from build123d import *

# Parameters (mm, degrees)
F0_W      = 78.3574953675
F0_H      = 53.3467046916
F1_DEPTH  = 50.8
F3_DEPTH  = 50.801
F4_W      = 25.4
F4_H      = 40.6467046916
F5_DEPTH  = 50.801
F6_W      = 12.7
F6_H      = 12.7
F7_DEPTH  = 50.801
F9_DEPTH  = 12.7
F11_DEPTH = 12.7
F13_DEPTH = 78.3584953675
F14_R     = 6.35


with BuildPart() as f1:
    # F0 (on Front) → F1 (new body)
    with BuildSketch(Plane.XZ):
        with Locations((39.1787476838, 26.6733523458)):
            Rectangle(F0_W, F0_H)
    extrude(amount=-F1_DEPTH)

    # F2 (on face) → F3 (cut, through all)
    with BuildSketch(Plane.XZ):
        Polygon((0, 53.3467046916), (0, 40.6467046916), (12.7, 53.3467046916), align=None)
    extrude(amount=-F3_DEPTH, mode=Mode.SUBTRACT)

    # F4 (on face) → F5 (cut, through all)
    with BuildSketch(Plane.XZ):
        with Locations((65.6574953675, 33.0233523458)):
            Rectangle(F4_W, F4_H)
    extrude(amount=-F5_DEPTH, mode=Mode.SUBTRACT)

    # F6 (on face) → F7 (cut, through all)
    with BuildSketch(Plane.XZ):
        with Locations((46.6074953675, 46.9967046916)):
            Rectangle(F6_W, F6_H)
    extrude(amount=-F7_DEPTH, mode=Mode.SUBTRACT)

    # F8 (on face) → F9 (cut)
    with BuildSketch(Plane.XZ):
        Polygon((27.5574953675, 27.9467046916), (52.9574953675, 27.9467046916), (52.9574953675, 40.6467046916), (40.2574953675, 40.6467046916), (40.2574953675, 53.3467046916), (27.5574953675, 53.3467046916), align=None)
    extrude(amount=-F9_DEPTH, mode=Mode.SUBTRACT)

    # F10 (on face) → F11 (cut)
    with BuildSketch(Plane(origin=(0, 50.8, 0), x_dir=(-1, 0, 0), z_dir=(0, 1, 0))):
        Polygon((-52.9574953675, 40.6467046916), (-52.9574953675, 27.9467046916), (-27.5574953675, 27.9467046916), (-27.5574953675, 53.3467046916), (-40.2574953675, 53.3467046916), (-40.2574953675, 40.6467046916), align=None)
    extrude(amount=-F11_DEPTH, mode=Mode.SUBTRACT)

    # F12 (on face) → F13 (cut, through all)
    with BuildSketch(Plane.YZ.offset(78.3574953675)):
        with BuildLine():
            ThreePointArc((19.05, 12.7), (25.4, 6.35), (31.75, 12.7))
            Line((31.75, 12.7), (19.05, 12.7))
        make_face()
        with BuildLine():
            Line((19.05, 12.7), (31.75, 12.7))
            ThreePointArc((31.75, 12.7), (25.4, 19.05), (19.05, 12.7))
        make_face()
    extrude(amount=-F13_DEPTH, mode=Mode.SUBTRACT)

    # F14
    f14_edges = [f1.edges().sort_by_distance(p)[0] for p in [
        (78.357495, 50.8, 6.35),
        (78.357495, 0, 6.35),
    ]]
    fillet(f14_edges, radius=F14_R)


solid = f1.part
Verification items for the finished model (mm, model axes). A direction names the side the tool comes from. Coordinates: 2 decimals unless noted, no trailing zeros. Order: outer loops, then holes, each group sorted by start corner. A loop starts at its lowest first (then second) coordinate and runs counter-clockwise, first axis right, second up. Notation, with made-up numbers: M 35.25,11 L 61.25,11 A23 cw 61.25,27 Z; hole C -29.5,76.25 d5. An arc over 180 degrees is marked long. Write each question's results on one line, items separated by ' | '.
1) Scan lines: line 1 along Z through (x, y) = (43, 25.4); line 2 along Y through (x, z) = (25.5, 12.7); line 3 along Z through (x, y) = (17, 25.4). Record each from-to range of solid material in increasing order. Write a range as [from, to].
Solved:
line 1: z = [0, 6.35], [19.05, 40.65] | line 2: y = [0, 19.05], [31.75, 50.8] | line 3: z = [0, 6.35], [19.05, 53.35]
2) Gauge pin test, flat ends, axial feed: pin 1 Ø12.5 at (x, z) = (44, 38.5) entering from -Y; pin 2 Ø2 at (y, z) = (41.5, 39.5) entering from +X; pin 3 Ø21 at (x, y) = (71.5, 36.5) entering from +Z. Record the tip position at first contact, or that the pin passes through.
Solved:
pin 1: stops at y = 12.7 | pin 2: stops at x = 27.56 | pin 3: stops at z = 12.7
3) Access from +Z, -Z, +X, -X, +Y, -Y to the whole of each face (thin tool, end or side, straight path). Record for faces 1 (the face through (40, 6, 27.947)), 2 (the face through (47, 25, 40.647)), 3 (the face through (27.557, 45, 40)).
Solved:
face 1: +Z, +X, -Y | face 2: +Z, +X, +Y, -Y | face 3: +Z, +X, +Y
4) Release check for a two-part mould opening along Y. For faces 4 (the face through (31.02, 24.02, 6.5)), 5 (the face through (38, 38.1, 38)), 6 (the face through (65, 41, 12.7)) record: pulls with the +Y half, pulls with the -Y half, needs draft (parallel to the pull), parting line crosses it, or undercut.
Solved:
face 4: undercut | face 5: pulls with the +Y half | face 6: needs draft
5) Section check D-D on y = 42.5. Record the cut outline in (x, z), plus the area to 3 significant figures.
Solved:
outline: M 0,0 L 78.36,0 L 78.36,12.7 L 52.96,12.7 L 52.96,27.95 L 27.56,27.95 L 27.56,53.35 L 12.7,53.35 L 0,40.65 Z | area: 2,420 mm²
6) Section check C-C on z = 29. Record the cut outline in (x, y), plus the area to 3 significant figures.
Solved:
outline: M 0,0 L 27.56,0 L 27.56,12.7 L 52.96,12.7 L 52.96,38.1 L 27.56,38.1 L 27.56,50.8 L 0,50.8 Z | area: 2,050 mm²
7) Section check B-B on x = 28.5. Record the cut outline in (y, z), plus the area to 3 significant figures.
Solved:
outline: M 0,0 L 50.8,0 L 50.8,27.95 L 38.1,27.95 L 38.1,53.35 L 12.7,53.35 L 12.7,27.95 L 0,27.95 Z; hole C 25.4,12.7 d12.7 | area: 1,940 mm²
8) Section check A-A on y = 25.4. Record the cut outline in (x, z).
Solved:
outline: M 0,0 L 78.36,0 L 78.36,6.35 L 0,6.35 Z; M 0,19.05 L 52.96,19.05 L 52.96,40.65 L 40.26,40.65 L 40.26,53.35 L 12.7,53.35 L 0,40.65 Z
